Part print with two shaded views. Sizes in mm from the minimum x, y, z corner. Round coordinates to 2 decimals unless told otherwise and drop trailing zeros. Order: outer loops, then holes, each group sorted by start corner. A loop starts at its lowest first (then second) coordinate and runs counter-clockwise, first axis right, second up. Notation, with made-up numbers: (71, -7) -> (123, -7) arc R11 ccw to (123, 5) -> close; hole circle Ø6 at (-2, -34). An arc over 180 degrees is marked (long way). Put each result on its own line as item: value. Start each with the question number.
Q1. Cut at D-D, the plane z = 123.5. List the corners of the cut face in (x, y).
Q2. Flat gauge pins, fed straight in: P1, Ø2.5, axis at x = 92.5, y = 3, coming from the -Z side; P2, Ø1.4, axis at x = 108.5, y = 1.5, coming from the +Z side; P3, Ø2.5, axis at y = 1.5, z = 183.5, coming from the -X side. Where does each tip first touch, or does it go through?
Q3. Probe L1, parallel to Z at x = 145, y = 4.55 (1 decimal); L2, parallel to Z at x = 135.5, y = 4.3 (1 decimal); L3, parallel to X at y = 0.95, z = 107 (1 decimal). List the from-to ranges inside material, lowest first.
Q4. Cut at B-B, the plane x = 104.5. List the corners of the cut face in (y, z).
Q5. Cut at C-C, the plane y = 3.8. State how many separate pieces and enclosed holes the cut face has, and give its area (3 significant figures).
Q6. Cut at A-A, the plane z = 34.5. List the corners of the cut face in (x, y).
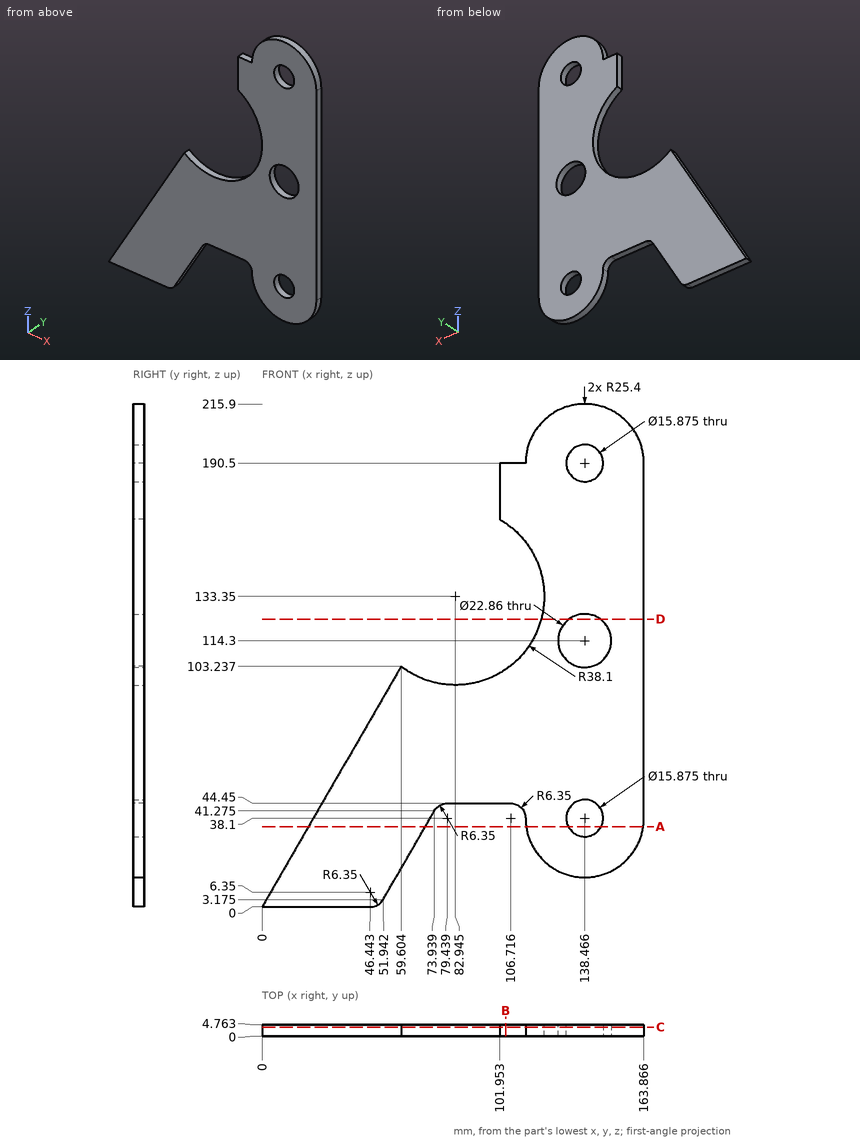
Ans:
1. outline: (119.75, 0) -> (131.68, 0) -> (131.68, 4.76) -> (119.75, 4.76) -> close; (145.25, 0) -> (163.87, 0) -> (163.87, 4.76) -> (145.25, 4.76) -> close
2. P1: stops at z = 44.45
2. P2: stops at z = 190.5
2. P3: stops at x = 101.95
3. L1: z = 13.6 to 33.6, 42.6 to 104.9, 123.7 to 186, 195 to 215
3. L2: z = 12.9 to 30.7, 45.5 to 103.3, 125.3 to 183.1, 197.9 to 215.7
3. L3: x = 110.5 to 129.7, 147.3 to 163.9
4. outline: (0, 44.45) -> (4.76, 44.45) -> (4.76, 101.93) -> (0, 101.93) -> close; (0, 164.77) -> (4.76, 164.77) -> (4.76, 190.5) -> (0, 190.5) -> close
5. separate pieces: 1
5. enclosed holes: 3
5. area: 15,200 mm^2
6. outline: (19.92, 0) -> (70.03, 0) -> (70.03, 4.76) -> (19.92, 4.76) -> close; (113.32, 0) -> (131.39, 0) -> (131.39, 4.76) -> (113.32, 4.76) -> close; (145.54, 0) -> (163.61, 0) -> (163.61, 4.76) -> (145.54, 4.76) -> close
